Read the model definition and answer for the solid it produces. Units are mm, in the model's axes. A direction names the side the tool comes from. Coordinates: 2 decimals unless noted, no trailing zeros. Order: outer loops, then holes, each group sorted by start corner. A loop starts at its lowest first (then second) coordinate and runs counter-clockwise, first axis right, second up. Notation, with made-up numbers: M 60,14 L 115,14 A32 cw 115,52 Z; hole C 44,48 d7. An arc over 180 degrees is marked long. One line per question, with ' | ' between items. Start each with the question number.
1) The mould has two halves that part along Y. Classify faces 4 (the face through (-10.8, 24.2, 2.5)), 5 (the face through (-5, 0, 2)), 6 (the face through (-13.88, 30.564, 3.979)): +Y half, -Y half, draft (parallel to the pull), parting line (faces both ways), or undercut.
2) Given P1, Ø4, axis at y = 17.5, z = -2, coming from the -X side; P2, Ø9, axis at x = 0, z = 0, coming from the +Y side; P3, Ø4, axis at x = -11.5, y = 12.5, coming from the -Z side; P4, Ø4, axis at y = 22, z = -6, coming from the -X side, each flat-ended and moving along its own axis, determine where each tip first touches the part or whether it passes through.
3) A tool of negligible diameter and unlimited length cuts with its end or side. For faces 1 (the face through (-16.764, 11.53, 5.035)), 2 (the face through (-8.1, 20.28, 1.93)), 3 (the face through (-11.08, 9.414, 3.979)), from which of +Z, -Z, +X, -X, +Y, -Y can it reach the whole face along a straight path? Write none if from no direction.
4) Consider probe 1 along Z at (x, y) = (0, 20) (3 decimals); probe 2 along Y at (x, z) = (-12.5, 6.65). Determine where each line is inside the solid, lowest interval first.
5) Find section A-A, the plane y = 33. Write down the section's boundary in (x, z) (3 decimals).
6) Find section D-D, the plane z = 4.5. Write down the section's boundary in (x, y).
7) Find section C-C, the plane y = 15.5. Write down the section's boundary in (x, z) (3 decimals).
8) Find section B-B, the plane x = -3.5. Write down the section's boundary in (y, z) (3 decimals).
from build123d import *

# Parameters (mm, degrees)
CROQUIS1_R              = 5.075
SALIENTE_EXTRUIR1_DEPTH = 40
CROQUIS2_R              = 1.6
CORTAR_EXTRUIR1_DEPTH   = 6
CORTAR_EXTRUIR2_DEPTH   = 3
CORTAR_EXTRUIR3_DEPTH   = 6
REDONDEO1_R             = 4
REDONDEO2_R             = 2


with BuildPart() as part:
    # Croquis1 → Saliente-Extruir1 (new body)
    with BuildSketch(Plane(origin=(0, 0, 0), x_dir=(1, 0, 0), z_dir=(0, 1, 0))):
        with BuildLine():
            Line((-17.5, -7.5), (7.5, -7.5))
            Line((7.5, -7.5), (7.5, 0))
            ThreePointArc((7.5, 0), (0, 7.5), (-7.5, 0))
            Line((-7.5, 0), (-7.5, -2.5))
            Line((-7.5, -2.5), (-17.5, -2.5))
            Line((-17.5, -2.5), (-17.5, -7.5))
        make_face()
        Circle(CROQUIS1_R, mode=Mode.SUBTRACT)
    extrude(amount=SALIENTE_EXTRUIR1_DEPTH)

    # Croquis2 → Cortar-Extruir1 (cut, through all)
    with BuildSketch(Plane(origin=(0, 0, 2.5), x_dir=(-1, 0, 0), z_dir=(0, 0, -1))):
        with Locations((12.5, 7)):
            Circle(CROQUIS2_R)
        with Locations((12.5, 33)):
            Circle(CROQUIS2_R)
    extrude(amount=-CORTAR_EXTRUIR1_DEPTH, mode=Mode.SUBTRACT)

    # Croquis3 → Cortar-Extruir2 (cut)
    with BuildSketch(Plane(origin=(0, 0, 2.5), x_dir=(-1, 0, 0), z_dir=(0, 0, -1))):
        Polygon((15.3, 31.383419246), (15.3, 34.616580754), (12.5, 36.233161507), (9.7, 34.616580754), (9.7, 31.383419246), (12.5, 29.766838493), align=None)
        Polygon((12.5, 10.233161507), (15.3, 8.616580754), (15.3, 5.383419246), (12.5, 3.766838493), (9.7, 5.383419246), (9.7, 8.616580754), align=None)
    extrude(amount=-CORTAR_EXTRUIR2_DEPTH, mode=Mode.SUBTRACT)

    # Croquis4 → Cortar-Extruir3 (cut, through all)
    with BuildSketch(Plane(origin=(0, 0, 2.5), x_dir=(-1, 0, 0), z_dir=(0, 0, -1))):
        with BuildLine():
            Line((17.5, 27.5), (17.5, 12.5))
            ThreePointArc((17.5, 12.5), (10, 20), (17.5, 27.5))
        make_face()
    extrude(amount=-CORTAR_EXTRUIR3_DEPTH, mode=Mode.SUBTRACT)

    # Redondeo1
    redondeo1_edges = [part.edges().sort_by_distance(p)[0] for p in [
        (-17.5, 40, 5),
        (-17.5, 12.5, 5),
        (-17.5, 27.5, 5),
        (-17.5, 0, 5),
    ]]
    fillet(redondeo1_edges, radius=REDONDEO1_R)

    # Redondeo2
    redondeo2_edges = [part.edges().sort_by_distance(p)[0] for p in [
        (-7.5, 20, 2.5),
        (7.5, 20, 7.5),
    ]]
    fillet(redondeo2_edges, radius=REDONDEO2_R)


solid = part.part
Report:
1) face 4: draft | face 5: -Y half | face 6: undercut
2) P1: stops at x = -7.5 | P2: passes through | P3: stops at z = 2.5 | P4: stops at x = -6.34
3) face 1: +Z, -Z, -X | face 2: -Z, -X, +Y, -Y | face 3: -Z
4) probe 1: z = -7.5 to -5.075, 5.075 to 7.5 | probe 2: y = 0 to 5.4, 8.6 to 14.41, 25.59 to 31.4, 34.6 to 40
5) outline: M -17.5,2.5 L -15.3,2.5 L -15.3,5.5 L -14.1,5.5 L -14.1,7.5 L -17.5,7.5 Z; M -10.9,5.5 L -9.7,5.5 L -9.7,2.5 L -9.5,2.5 A2 cw -7.5,0.5 L -7.5,0 A7.5 ccw 7.5,0 L 7.5,5.5 A2 ccw 5.5,7.5 L -10.9,7.5 Z; hole C 0,0 d10.15
6) outline: M -17.5,4 A4 ccw -13.5,0 L -2.35,0 L -2.35,40 L -13.5,40 A4 ccw -17.5,36 L -17.5,30.78 A4 ccw -14.89,27.03 A7.5 cw -14.89,12.97 A4 ccw -17.5,9.22 Z; M 2.35,0 L 7.5,0 L 7.5,40 L 2.35,40 Z; hole M -15.3,5.38 L -12.5,3.77 L -9.7,5.38 L -9.7,8.62 L -12.5,10.23 L -15.3,8.62 Z; hole M -15.3,31.38 L -12.5,29.77 L -9.7,31.38 L -9.7,34.62 L -12.5,36.23 L -15.3,34.62 Z
7) outline: M -11.5,2.5 L -9.5,2.5 A2 cw -7.5,0.5 L -7.5,0 A7.5 ccw 7.5,0 L 7.5,5.5 A2 ccw 5.5,7.5 L -11.5,7.5 Z; hole C 0,0 d10.15
8) outline: M 0,-6.633 L 40,-6.633 L 40,-3.675 L 0,-3.675 Z; M 0,3.675 L 40,3.675 L 40,7.5 L 0,7.5 Z
